Check sheet for the modelled part. Datum: model origin and axes. Units: mm. Face numbers are marked on the shaded views. Round coordinates to 2 decimals unless told otherwise and drop trailing zeros. Loops run counter-clockwise (first coordinate to the right, second up) from the corner with the lowest first, then second, coordinate; pieces in that order, holes last. Notation, with made-up numbers: (-35.5, 12.5) - (13.5, 12.5) arc R23 cw to (13.5, 24.5) - close; hole circle Ø2 at (27, -17.75). An arc over 180 degrees is marked (long way). Answer in a Markdown table with one row per item. Add a question column.
(1) Cross-section at A-A on x = 0. Enter the section's corners in (y, z), then the cut area to 3 significant figures.
(2) Mould release check, pull along X, two halves, no side actions. Record for the marked faces 1, 2 and 3: +X half, -X half, draft (parallel to the pull), parting line (faces both ways), or undercut.
(3) Gauge pin test, flat ends, axial feed: pin 1 (3 mm diameter, centred on y = 1, z = -1.5, fed in from -X); pin 2 (2 mm diameter, centred on x = 0.5, y = 1.5, fed in from +Z). Record the tip position at first contact, or that the pin passes through.
(4) Cross-section at C-C on y = 1.75. Enter the section's corners in (x, z).
(5) Thickness scan on line 1 along Z through (x, y) = (0, 1.7); line 2 along Z through (x, y) = (-1.5, 0.9). Record the ranges inside material, lowest first.
(6) Cross-section at B-B on z = 0. Enter the section's corners in (x, y), then the cut area to 3 significant figures.
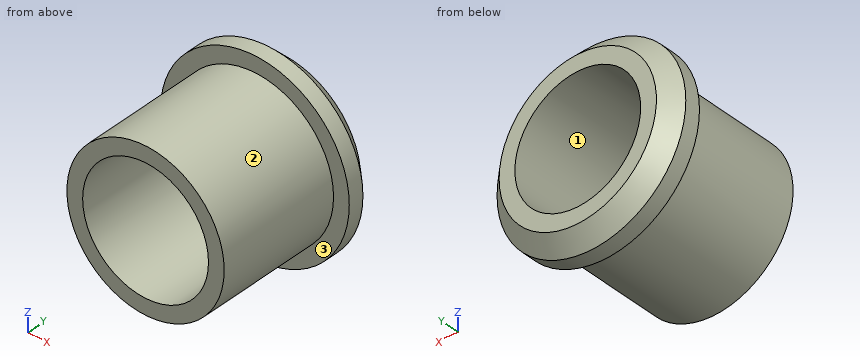
from build123d import *

# Parameters (mm, degrees)
SKETCH2_R           = 2.5
SKETCH2_R_2         = 2
BOSS_EXTRUDE1_DEPTH = 4
SKETCH3_R           = 3
SKETCH3_R_2         = 2
BOSS_EXTRUDE2_DEPTH = 1
CHAMFER1_SIZE       = 0.5


with BuildPart() as part:
    # Sketch2 → Boss-Extrude1 (new body)
    with BuildSketch(Plane(origin=(0, 0, 0), x_dir=(1, 0, 0), z_dir=(0, 1, 0))):
        Circle(SKETCH2_R)
        Circle(SKETCH2_R_2, mode=Mode.SUBTRACT)
    extrude(amount=BOSS_EXTRUDE1_DEPTH)

    # Sketch3 → Boss-Extrude2 (add)
    with BuildSketch(Plane(origin=(0, 4, 0), x_dir=(1, 0, 0), z_dir=(0, 1, 0))):
        Circle(SKETCH3_R)
        Circle(SKETCH3_R_2, mode=Mode.SUBTRACT)
    extrude(amount=BOSS_EXTRUDE2_DEPTH)

    # Chamfer1
    chamfer1_edges = [part.edges().sort_by_distance(p)[0] for p in [
        (-3, 5, 0),
    ]]
    chamfer(chamfer1_edges, length=CHAMFER1_SIZE)


solid = part.part
Answers:
| question | item | result |
|---|---|---|
| 1 | outline | (0, -2.5) - (4, -2.5) - (4, -3) - (4.5, -3) - (5, -2.5) - (5, -2) - (0, -2) - close; (0, 2) - (5, 2) - (5, 2.5) - (4.5, 3) - (4, 3) - (4, 2.5) - (0, 2.5) - close |
| 1 | area | 5.75 mm^2 |
| 2 | face 1 | undercut |
| 2 | face 2 | parting line |
| 2 | face 3 | draft |
| 3 | pin 1 | stops at x = -2.5 |
| 3 | pin 2 | stops at z = 2.5 |
| 4 | outline | circle Ø5 at (0, 0); hole circle Ø4 at (0, 0) |
| 5 | line 1 | z = -2.5 to -2, 2 to 2.5 |
| 5 | line 2 | z = -2 to -1.32, 1.32 to 2 |
| 6 | outline | (-3, 4) - (-2.5, 4) - (-2.5, 0) - (-2, 0) - (-2, 5) - (-2.5, 5) - (-3, 4.5) - close; (2, 0) - (2.5, 0) - (2.5, 4) - (3, 4) - (3, 4.5) - (2.5, 5) - (2, 5) - close |
| 6 | area | 5.75 mm^2 |
